```python
from build123d import *

# Parameters (mm, degrees)
F0_R     = 14.2875
F0_W     = 149.225
F0_H     = 149.225
F1_DEPTH = 15.875
F2_START = 9.525
F0_R_2   = 36.5125
F2_DEPTH = 6.35


with BuildPart() as f1:
    # F0 (on Front) → F1 (new body)
    with BuildSketch(Plane.XZ):
        Polygon((609.6, 0), (-609.6, 0), (-609.6, -406.4), (-406.4, -609.5745491936), (406.4, -609.5745491936), (609.6, -406.4), align=None)
        with Locations((-355.6, -427.0120491936)):
            Circle(F0_R, mode=Mode.SUBTRACT)
        with Locations((-415.2417373546, -326.1154076089)):
            Circle(F0_R, mode=Mode.SUBTRACT)
        with Locations((-260.35, -444.4745491936)):
            Circle(F0_R, mode=Mode.SUBTRACT)
        with Locations((-222.25, -444.4745491936)):
            Circle(F0_R, mode=Mode.SUBTRACT)
        with Locations((-184.15, -444.4745491936)):
            Circle(F0_R, mode=Mode.SUBTRACT)
        with Locations((-260.35, -409.5495491936)):
            Circle(F0_R, mode=Mode.SUBTRACT)
        with Locations((-222.25, -409.5495491936)):
            Circle(F0_R, mode=Mode.SUBTRACT)
        with Locations((-184.15, -409.5495491936)):
            Circle(F0_R, mode=Mode.SUBTRACT)
        with Locations((184.15, -427.0120491936)):
            Circle(F0_R, mode=Mode.SUBTRACT)
        with Locations((279.4, -444.4745491936)):
            Circle(F0_R, mode=Mode.SUBTRACT)
        with Locations((279.4, -409.5495491936)):
            Circle(F0_R, mode=Mode.SUBTRACT)
        with Locations((0, -355.5745491936)):
            Rectangle(F0_W, F0_H, mode=Mode.SUBTRACT)
        with Locations((317.5, -444.4745491936)):
            Circle(F0_R, mode=Mode.SUBTRACT)
        with Locations((355.6, -444.4745491936)):
            Circle(F0_R, mode=Mode.SUBTRACT)
        with Locations((317.5, -409.5495491936)):
            Circle(F0_R, mode=Mode.SUBTRACT)
        with Locations((355.6, -409.5495491936)):
            Circle(F0_R, mode=Mode.SUBTRACT)
        with Locations((400.4724875181, -309.6562085607)):
            Circle(F0_R, mode=Mode.SUBTRACT)
        with Locations((-508, -228.6)):
            Circle(F0_R, mode=Mode.SUBTRACT)
        with Locations((-444.5, -301.7112262669)):
            Circle(F0_R, mode=Mode.SUBTRACT)
        with Locations((-393.4358199474, -298.8343227509)):
            Circle(F0_R, mode=Mode.SUBTRACT)
        with Locations((-422.6940825928, -274.4301414089)):
            Circle(F0_R, mode=Mode.SUBTRACT)
        with Locations((-438.15, -76.2)):
            Circle(F0_R, mode=Mode.SUBTRACT)
        with Locations((-400.05, -76.2)):
            Circle(F0_R, mode=Mode.SUBTRACT)
        with Locations((-247.65, -76.2)):
            Circle(F0_R, mode=Mode.SUBTRACT)
        with Locations((-209.55, -76.2)):
            Circle(F0_R, mode=Mode.SUBTRACT)
        with Locations((-57.15, -76.2)):
            Circle(F0_R, mode=Mode.SUBTRACT)
        with Locations((-19.05, -76.2)):
            Circle(F0_R, mode=Mode.SUBTRACT)
        with Locations((456.4161513597, -230.8944980995)):
            Circle(F0_R, mode=Mode.SUBTRACT)
        with Locations((481.1103089784, -255.5917490498)):
            Circle(F0_R, mode=Mode.SUBTRACT)
        with Locations((508, -228.6)):
            Circle(F0_R, mode=Mode.SUBTRACT)
        with Locations((483.3058423812, -203.9027490498)):
            Circle(F0_R, mode=Mode.SUBTRACT)
        with Locations((19.05, -76.2)):
            Circle(F0_R, mode=Mode.SUBTRACT)
        with Locations((57.15, -76.2)):
            Circle(F0_R, mode=Mode.SUBTRACT)
        with Locations((209.55, -76.2)):
            Circle(F0_R, mode=Mode.SUBTRACT)
        with Locations((247.65, -76.2)):
            Circle(F0_R, mode=Mode.SUBTRACT)
        with Locations((400.05, -76.2)):
            Circle(F0_R, mode=Mode.SUBTRACT)
        with Locations((438.15, -76.2)):
            Circle(F0_R, mode=Mode.SUBTRACT)
    extrude(amount=F1_DEPTH)

    # F0 (on Front) → F2 (join)
    with BuildSketch(Plane.XZ.offset(F2_START)):
        with Locations((0, -355.5745491936)):
            Rectangle(F0_W, F0_H)
        with Locations((0, -355.5745491936)):
            Circle(F0_R_2, mode=Mode.SUBTRACT)
    extrude(amount=F2_DEPTH)


solid = f1.part
```
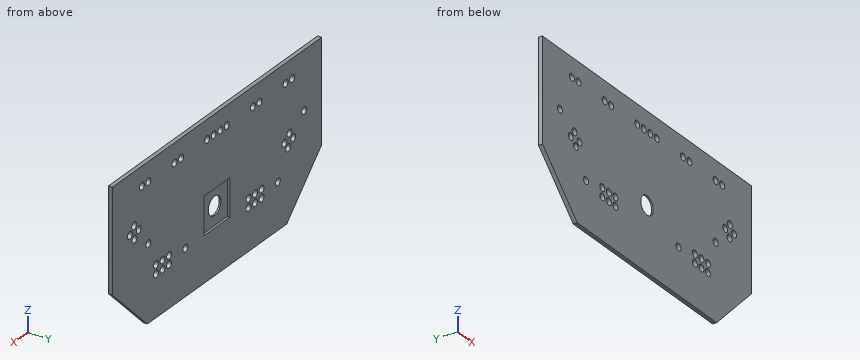
Design review of the part built by this model. Coordinates are the model's own, in mm. Coordinates: 2 decimals unless noted, no trailing zeros. Order: outer loops, then holes, each group sorted by start corner. A loop starts at its lowest first (then second) coordinate and runs counter-clockwise, first axis right, second up.
1) Take a section at B-B, the plane x = -57.15. Give the boundary of the cut face in (y, z) (1 decimal), and give its area (3 significant figures).
2) Take a section at A-A, the plane x = 279.4. Give the boundary of the cut face in (y, z) (3 decimals).
3) Take a section at D-D, the plane y = -2.5. State how many separate pieces and enclosed holes the cut face has, and give its area (3 significant figures).
4) Wall thickness on line 1 along Z through (x, y) = (400.05, -11.25); line 2 along Z through (x, y) = (357, -11.75); line 3 along Z through (x, y) = (183, -4.75): over which ranges is each line inside the solid? List them lowest first.
5) Take a section at C-C, the plane z = -488. Give the boundary of the cut face in (x, y) (3 decimals).
6) Clearance check with flat-ended pins moving along their axes: pin 1 (4 mm diameter, centred on x = -486, y = -14, fed in from -Z); pin 2 (4 mm diameter, centred on x = -467, y = -7, fed in from -Z); pin 3 (1 mm diameter, centred on x = -481.5, y = -13, fed in from -Z); pin 4 (8 mm diameter, centred on x = 76.5, y = -11, fed in from +Z). State where each tip first meets the part, or that it passes through.
Returned:
1. outline: (-15.9, -609.6) - (0, -609.6) - (0, -430.2) - (-9.5, -430.2) - (-9.5, -281) - (0, -281) - (0, -90.5) - (-15.9, -90.5) - close; (-15.9, -61.9) - (0, -61.9) - (0, 0) - (-15.9, 0) - close
1. area: 7,800 mm2
2. outline: (-15.875, -609.575) - (0, -609.575) - (0, -458.762) - (-15.875, -458.762) - close; (-15.875, -430.187) - (0, -430.187) - (0, -423.837) - (-15.875, -423.837) - close; (-15.875, -395.262) - (0, -395.262) - (0, 0) - (-15.875, 0) - close
3. separate pieces: 1
3. enclosed holes: 37
3. area: 657,000 mm2
4. line 1: z = -609.57 to -323.94, -295.37 to -90.49, -61.91 to 0
4. line 2: z = -609.57 to -458.69, -430.26 to -423.77, -395.33 to 0
4. line 3: z = -609.57 to -441.25, -412.77 to 0
5. outline: (-527.99, -15.875) - (527.99, -15.875) - (527.99, 0) - (-527.99, 0) - close
6. pin 1: stops at z = -531.98
6. pin 2: stops at z = -550.98
6. pin 3: stops at z = -534.98
6. pin 4: stops at z = 0
